Model file for the job. Use its own axes, mm. Round coordinates to 2 decimals unless told otherwise and drop trailing zeros. Loops run counter-clockwise (first coordinate to the right, second up) from the corner with the lowest first, then second, coordinate; pieces in that order, holes last. Notation, with made-up numbers: M 61,-29 L 106,-29 A31 ccw 106,4 Z; hole C -24,19 d5. An arc over 180 degrees is marked long. Use a Markdown table: item, result. Add a question column.
Q1. Probe line 1 (X direction, y = -234, z = 0.55); line 2 (Y direction, x = 12, z = 1.35); line 3 (X direction, y = -147.5, z = 1.9). List the from-to ranges inside material, lowest first. Write a range as from..to.
Q2. Cut at C-C (x = 12). Give the cut face in (y, z), plus the area to 3 significant figures.
Q3. Cut at A-A (y = -247.5). Give the cut face in (x, z).
Q4. Pin check, flat tips, straight feed: pin 1 (1 mm diameter, centred on x = -1, z = 1.5, fed in from +Y); pin 2 (3 mm diameter, centred on x = 32.5, y = -194.55, fed in from +Z); pin 3 (0.6 mm diameter, centred on x = 6.5, z = 1.5, fed in from +Y); pin 4 (1 mm diameter, centred on y = -231.5, z = 1, fed in from -X). Stop position of each tip, or through.
Q5. Cut at B-B (x = 32.5). Give the cut face in (y, z).
Q6. Cut at D-D (y = -167.5). Give the cut face in (x, z).
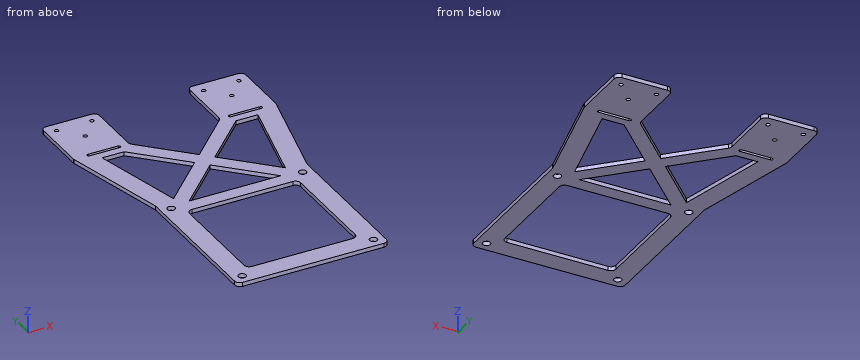
from build123d import *

# Parameters (mm, degrees)
SKETCH1_R           = 1.875
SKETCH1_R_2         = 1
BOSS_EXTRUDE2_DEPTH = 2


with BuildPart() as part:
    # Sketch1 → Boss-Extrude2 (new body)
    with BuildSketch(Plane.XY):
        with BuildLine():
            Line((-35, -264.548366883), (35, -264.548366883))
            ThreePointArc((35, -264.548366883), (36.767766953, -263.816133836), (37.5, -262.048366883))
            Line((37.5, -262.048366883), (37.5, -189.844720828))
            ThreePointArc((37.5, -189.844720828), (37.517382153, -189.550427391), (37.569286901, -189.260226318))
            Line((37.569286901, -189.260226318), (49.928636869, -137.861909768))
            ThreePointArc((49.928636869, -137.861909768), (49.980541617, -137.571708695), (49.99792377, -137.277415258))
            Line((49.99792377, -137.277415258), (49.99792377, -110.073769203))
            ThreePointArc((49.99792377, -110.073769203), (49.265690723, -108.30600225), (47.49792377, -107.573769203))
            Line((47.49792377, -107.573769203), (24.98250936, -107.573769203))
            ThreePointArc((24.98250936, -107.573769203), (23.214742407, -108.30600225), (22.48250936, -110.073769203))
            Line((22.48250936, -110.073769203), (22.48250936, -136.538235297))
            ThreePointArc((22.48250936, -136.538235297), (22.292208191, -137.494943878), (21.750276313, -138.30600225))
            Line((21.750276313, -138.30600225), (0.000286917, -160.055991645))
            Line((0.000286917, -160.055991645), (-21.749702478, -138.30600225))
            ThreePointArc((-21.749702478, -138.30600225), (-22.291634357, -137.494943878), (-22.481935525, -136.538235297))
            Line((-22.481935525, -136.538235297), (-22.481935525, -110.073769203))
            ThreePointArc((-22.481935525, -110.073769203), (-23.214168572, -108.30600225), (-24.981935525, -107.573769203))
            Line((-24.981935525, -107.573769203), (-47.49792377, -107.573769203))
            ThreePointArc((-47.49792377, -107.573769203), (-49.265690723, -108.30600225), (-49.99792377, -110.073769203))
            Line((-49.99792377, -110.073769203), (-49.99792377, -137.277415258))
            ThreePointArc((-49.99792377, -137.277415258), (-49.980541617, -137.571708695), (-49.928636869, -137.861909768))
            Line((-49.928636869, -137.861909768), (-37.5, -189.548366883))
            Line((-37.5, -189.548366883), (-37.5, -262.048366883))
            ThreePointArc((-37.5, -262.048366883), (-36.767766953, -263.816133836), (-35, -264.548366883))
        make_face()
        with Locations((32.5, -259.548366883)):
            Circle(SKETCH1_R, mode=Mode.SUBTRACT)
        with Locations((-32.5, -259.548366883)):
            Circle(SKETCH1_R, mode=Mode.SUBTRACT)
        with Locations((-32.5, -194.548366883)):
            Circle(SKETCH1_R, mode=Mode.SUBTRACT)
        with Locations((32.5, -194.548366883)):
            Circle(SKETCH1_R, mode=Mode.SUBTRACT)
        with Locations((-45, -112.573769203)):
            Circle(SKETCH1_R_2, mode=Mode.SUBTRACT)
        with Locations((-27.481935525, -112.573769203)):
            Circle(SKETCH1_R_2, mode=Mode.SUBTRACT)
        with Locations((27.481935525, -113.029421113)):
            Circle(SKETCH1_R_2, mode=Mode.SUBTRACT)
        with Locations((45, -113.029421113)):
            Circle(SKETCH1_R_2, mode=Mode.SUBTRACT)
        with Locations((-36.239929648, -122.573769203)):
            Circle(SKETCH1_R_2, mode=Mode.SUBTRACT)
        with Locations((36.239929648, -122.573769203)):
            Circle(SKETCH1_R_2, mode=Mode.SUBTRACT)
        Polygon((-27.65637254, -187.712651103), (-38.552510863, -142.399332188), (-27.65637254, -142.399332188), (-4.999713083, -165.055991645), align=None, mode=Mode.SUBTRACT)
        Polygon((38.552510863, -142.399332188), (27.656946375, -187.712651103), (5.000286917, -165.055991645), (27.65637254, -142.399332188), align=None, mode=Mode.SUBTRACT)
        with BuildLine():
            Line((-27.5, -204.548366883), (-27.5, -249.548366883))
            Line((-27.5, -249.548366883), (-27.5, -252.048366883))
            ThreePointArc((-27.5, -252.048366883), (-26.767766953, -253.816133836), (-25, -254.548366883))
            Line((-25, -254.548366883), (-16.464466094, -254.548366883))
            Line((-16.464466094, -254.548366883), (16.464466094, -254.548366883))
            Line((16.464466094, -254.548366883), (25, -254.548366883))
            ThreePointArc((25, -254.548366883), (26.767766953, -253.816133836), (27.5, -252.048366883))
            Line((27.5, -252.048366883), (27.5, -249.548366883))
            Line((27.5, -249.548366883), (27.5, -204.548366883))
            Line((27.5, -204.548366883), (27.5, -202.048366883))
            ThreePointArc((27.5, -202.048366883), (26.767766953, -200.28059993), (25, -199.548366883))
            Line((25, -199.548366883), (22.5, -199.548366883))
            Line((22.5, -199.548366883), (-22.5, -199.548366883))
            Line((-22.5, -199.548366883), (-25, -199.548366883))
            ThreePointArc((-25, -199.548366883), (-26.767766953, -200.28059993), (-27.5, -202.048366883))
            Line((-27.5, -202.048366883), (-27.5, -204.548366883))
        make_face(mode=Mode.SUBTRACT)
        Polygon((-22.65637254, -192.712651103), (22.656946375, -192.712651103), (0.000286917, -170.055991645), align=None, mode=Mode.SUBTRACT)
        with BuildLine():
            Line((-42.587811549, -136.823769203), (-27.481935525, -136.823769203))
            ThreePointArc((-27.481935525, -136.823769203), (-26.731935525, -137.573769203), (-27.481935525, -138.323769203))
            Line((-27.481935525, -138.323769203), (-42.587811549, -138.323769203))
            ThreePointArc((-42.587811549, -138.323769203), (-43.337811549, -137.573769203), (-42.587811549, -136.823769203))
        make_face(mode=Mode.SUBTRACT)
        with BuildLine():
            Line((42.587811549, -136.823769203), (27.481935525, -136.823769203))
            ThreePointArc((27.481935525, -136.823769203), (26.731935525, -137.573769203), (27.481935525, -138.323769203))
            Line((27.481935525, -138.323769203), (42.587811549, -138.323769203))
            ThreePointArc((42.587811549, -138.323769203), (43.337811549, -137.573769203), (42.587811549, -136.823769203))
        make_face(mode=Mode.SUBTRACT)
    extrude(amount=BOSS_EXTRUDE2_DEPTH)


solid = part.part
Checked values:
| question | item | result |
|---|---|---|
| 1 | line 1 | x = -37.5..-27.5, 27.5..37.5 |
| 1 | line 2 | y = -264.55..-254.55, -199.55..-192.71, -182.06..-172.06, -158.06..-148.06 |
| 1 | line 3 | x = -47.61..-37.33, -22.56..-12.56, 12.56..22.56, 37.33..47.61 |
| 2 | outline | M -264.55,0 L -254.55,0 L -254.55,2 L -264.55,2 Z; M -199.55,0 L -192.71,0 L -192.71,2 L -199.55,2 Z; M -182.06,0 L -172.06,0 L -172.06,2 L -182.06,2 Z; M -158.06,0 L -148.06,0 L -148.06,2 L -158.06,2 Z |
| 2 | area | 73.7 mm^2 |
| 3 | outline | M -37.5,0 L -27.5,0 L -27.5,2 L -37.5,2 Z; M 27.5,0 L 37.5,0 L 37.5,2 L 27.5,2 Z |
| 4 | pin 1 | stops at y = -158.56 |
| 4 | pin 2 | passes through |
| 4 | pin 3 | stops at y = -153.26 |
| 4 | pin 4 | stops at x = -37.5 |
| 5 | outline | M -264.55,0 L -261.42,0 L -261.42,2 L -264.55,2 Z; M -257.67,0 L -196.42,0 L -196.42,2 L -257.67,2 Z; M -192.67,0 L -167.57,0 L -167.57,2 L -192.67,2 Z; M -142.4,0 L -138.32,0 L -138.32,2 L -142.4,2 Z; M -136.82,0 L -107.57,0 L -107.57,2 L -136.82,2 Z |
| 6 | outline | M -42.8,0 L -32.52,0 L -32.52,2 L -42.8,2 Z; M -7.44,0 L 7.44,0 L 7.44,2 L -7.44,2 Z; M 32.52,0 L 42.8,0 L 42.8,2 L 32.52,2 Z |
